Here's how the part is built. I have some questions about the finished solid (model axes, mm). Give positions to 0.01 mm unless a question says otherwise; leave off trailing zeros. Write each loop counter-clockwise with the first axis right and the second up, starting at its lowest first coordinate (ties: lowest second). Pieces come first, ordered by that corner, then holes. Notation, with made-up numbers: (65, 38.5) -> (85, 38.5) arc R24 ccw to (85, 70.5) -> close; hole circle Ø9 at (81.5, 16). An arc over 180 degrees is marked (long way). Return JSON: item names as keys, results as strings.
from build123d import *

# Parameters (mm, degrees)
SKETCH_1_R      = 6.05
SKETCH_1_R_2    = 6.1
SKETCH_1_R_3    = 3.05
SKETCH_1_R_4    = 3.25
EXTRUDE_1_DEPTH = 2


with BuildPart() as part:
    # 草图1 → 凸台-拉伸1 (new body)
    with BuildSketch(Plane(origin=(0, 0, 0), x_dir=(0, 0, -1), z_dir=(1, 0, 0))):
        with BuildLine():
            Line((19.426316451, -58.647367097), (-125.573683549, -58.647367097))
            ThreePointArc((-125.573683549, -58.647367097), (-150.573683549, -33.647367097), (-125.573683549, -8.647367097))
            Line((-125.573683549, -8.647367097), (4.992559722, -8.647367097))
            Line((4.992559722, -8.647367097), (19.426316451, -8.647367097))
            ThreePointArc((19.426316451, -8.647367097), (44.426316451, -33.647367097), (19.426316451, -58.647367097))
        make_face()
        with Locations((19.426316451, -33.647367097)):
            Circle(SKETCH_1_R, mode=Mode.SUBTRACT)
        with Locations((-125.573683549, -33.647367097)):
            Circle(SKETCH_1_R_2, mode=Mode.SUBTRACT)
        with Locations((-56.921571535, -43.647367097)):
            Circle(SKETCH_1_R_3, mode=Mode.SUBTRACT)
        with Locations((-15.573683549, -15.647367097)):
            Circle(SKETCH_1_R_4, mode=Mode.SUBTRACT)
        with Locations((-55.573683549, -15.647367097)):
            Circle(SKETCH_1_R_4, mode=Mode.SUBTRACT)
    extrude(amount=EXTRUDE_1_DEPTH)


solid = part.part
1. Suppose I cut it at C-C, the plane x = 1.35. List the corners of the cut face in (y, z) for me, and give its area (3 significant figures).
Taken from the geometry:
{"outline": "(-58.65, -19.43) arc R25 ccw to (-8.65, -19.43) -> (-8.65, 125.57) arc R25 ccw to (-58.65, 125.57) -> close; hole circle Ø6.1 at (-43.65, 56.92); hole circle Ø12.2 at (-33.65, 125.57); hole circle Ø12.1 at (-33.65, -19.43); hole circle Ø6.5 at (-15.65, 15.57); hole circle Ø6.5 at (-15.65, 55.57)", "area": "8,890 mm²"}
2. If I drill on line 1 (Z direction, x = 0.7, y = -33.5); line 2 (Z direction, x = 0.3, y = -30); line 3 (Y direction, x = 1.7, z = 55), over which ranges is the centre line in solid material (lowest first)? Write a range as [from, to].
Taken from the geometry:
{"line 1": "z = [-44.43, -25.47], [-13.38, 119.48], [131.67, 150.57]", "line 2": "z = [-44.16, -24.25], [-14.6, 120.68], [130.46, 150.31]", "line 3": "y = [-58.65, -46.02], [-41.28, -18.85], [-12.45, -8.65]"}
3. Suppose I cut it at D-D, the plane z = 57. List the corners of the cut face in (x, y) for me.
Taken from the geometry:
{"outline": "(0, -58.65) -> (2, -58.65) -> (2, -46.7) -> (0, -46.7) -> close; (0, -40.6) -> (2, -40.6) -> (2, -18.57) -> (0, -18.57) -> close; (0, -12.73) -> (2, -12.73) -> (2, -8.65) -> (0, -8.65) -> close"}
4. Suppose I cut it at B-B, the plane y = -37. List the corners of the cut face in (x, z) for me.
Taken from the geometry:
{"outline": "(0, -44.2) -> (2, -44.2) -> (2, -24.46) -> (0, -24.46) -> close; (0, -14.39) -> (2, -14.39) -> (2, 120.48) -> (0, 120.48) -> close; (0, 130.67) -> (2, 130.67) -> (2, 150.35) -> (0, 150.35) -> close"}
5. If we mould it in two halves opening along Y, with no side actions, what happens to faces 1 (the face through (2, -33, 52)), 2 (the face through (0.986, -17.625, 58.153)), 3 (the face through (0.99, -33.1, -44.42))? For each: released by +Y, released by -Y, zero draft, split by the parting line, or undercut.
Taken from the geometry:
{"face 1": "zero draft", "face 2": "undercut", "face 3": "split by the parting line"}
6. For pin 1 Ø3.5 at (y, z) = (-43.65, 56.92) entering from +X; pin 2 Ø1 at (x, y) = (1.5, -41) entering from +Z, each with a flat end and sliding along its axis, tell me the tip position at first contact or that it passes through.
Taken from the geometry:
{"pin 1": "passes through", "pin 2": "stops at z = 149.62"}
7. Suppose I cut it at A-A, the plane z = -16. List the corners of the cut face in (x, y) for me.
Taken from the geometry:
{"outline": "(0, -58.65) -> (2, -58.65) -> (2, -38.63) -> (0, -38.63) -> close; (0, -28.66) -> (2, -28.66) -> (2, -8.65) -> (0, -8.65) -> close"}
